Autodesk Inventor part; units mm, degrees
ref_plane "YZ Plane" through (0, 0, 0) normal (1, 0, 0) x (0, 1, 0)
ref_plane "XZ Plane" through (0, 0, 0) normal (0, 1, 0) x (-1, 0, 0)
ref_plane "XY Plane" through (0, 0, 0) normal (0, 0, 1) x (1, 0, 0)
sketch "Эскиз1" plane through (0, 0, 0) normal (1, 0, 0) x (0, 1, 0)
  circle A0 centre (0, 0) radius 7.5
  circle A1 centre (0, 0) radius 4
  dimension "d0" = 15
  dimension "d1" = 8
extrude "Выдавливание1" add sketch "Эскиз1" along normal mid plane 45
sketch "Эскиз2" plane through (22.5, 0, 0) normal (1, 0, 0) x (0, 0, -1)
  circle A0 centre (0, 0) radius 5
  circle A1 centre (0, 0) radius 6.5
  dimension "d4" = 10
  dimension "d5" = 13
extrude "Выдавливание2" cut sketch "Эскиз2" against normal blind 1
sketch "Эскиз3" plane through (-22.5, 0, 0) normal (-1, 0, 0) x (0, 0, 1)
  circle A0 centre (0, 0) radius 6.5
  circle A1 centre (0, 0) radius 5
  dimension "d9" = 13
  dimension "d10" = 10
extrude "Выдавливание3" cut sketch "Эскиз3" against normal blind 1
fillet "Сопряжение1" radius 0.5 1 edges at (-22.5, -7.5, 0)
fillet "Сопряжение2" radius 0.5 3 edges at (-22.5, -4, 0) (22.5, -7.5, 0) (22.5, -4, 0)
chamfer "Фаска1" distance 0.2 angle 45 8 edges at (22.5, 0, 5) (22.5, 0, 6.5) (-22.5, 0, -5) (-22.5, 0, -6.5) (-21.5, 0, -5) (-21.5, 0, -6.5) (21.5, 0, 6.5) (21.5, 0, 5)
properties part number "LM8LUU"
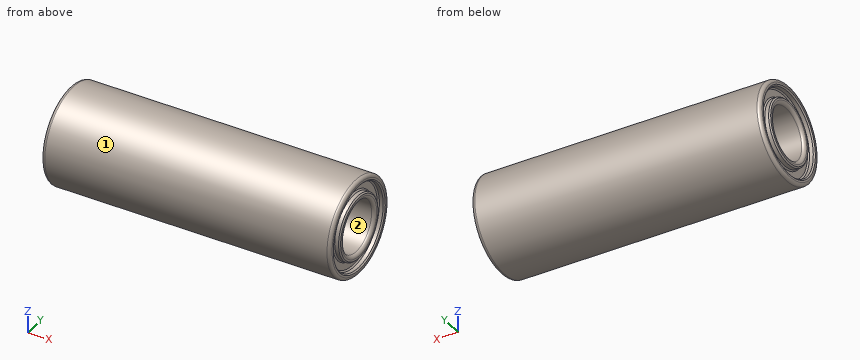
For this review, take the finished solid that the model builds, in its own axes (mm). Face numbers are marked on the shaded views. Round coordinates to 2 decimals unless told otherwise and drop trailing zeros. Loops run counter-clockwise (first coordinate to the right, second up) from the corner with the lowest first, then second, coordinate; pieces in that order, holes last. Notation, with made-up numbers: (42, 49.5) - (98, 49.5) arc R16 cw to (98, 73.5) - close; hole circle Ø4 at (-1.5, -3.5). An arc over 180 degrees is marked (long way). Use one line per item in the form item = value.
1) We need section A-A on x = -18.5. Write out the cut boundary in (y, z), then the cut area to 3 significant figures.
Solutions:
outline = circle Ø15 at (0, 0); hole circle Ø8 at (0, 0)
area = 126 mm2
2) Wall thickness on probe 1 along X at (y, z) = (-2.75, -6.5); probe 2 along Z at (x, y) = (-7, 0); probe 3 along Y at (x, z) = (-9, 0.5): over which ranges is each line inside the solid? List them lowest first.
Solutions:
probe_1 = -22.5 to 22.5
probe_2 = -7.5 to -4, 4 to 7.5
probe_3 = -7.48 to -3.97, 3.97 to 7.48
3) Mouldability with a two-part tool opening along Y and no side actions: class the marked faces 1 and 2 as pulls with the +Y half, pulls with the -Y half, needs draft (parallel to the pull), parting line crosses it, or undercut.
Solutions:
face_1 = parting line crosses it
face_2 = undercut
4) Clearance check with flat-ended pins moving along their axes: P1, Ø7, axis at y = 0, z = 0, coming from the -X side; P2, Ø1.5, axis at x = -14, y = 1.5, coming from the -Z side; P3, Ø6, axis at x = -13, z = 4.5, coming from the +Y side; P4, Ø1.5, axis at x = 12, z = 5, coming from the +Y side. State where each tip first meets the part, or that it passes through.
Solutions:
P1 = through
P2 = -7.46
P3 = 7.35
P4 = 6.18
